Geometry check sheet. Reference: the model listing, model coordinates, mm. A direction names the side the tool comes from. Round coordinates to 2 decimals unless told otherwise and drop trailing zeros. Write each loop counter-clockwise with the first axis right and the second up, starting at its lowest first coordinate (ties: lowest second). Pieces come first, ordered by that corner, then holes. Notation, with made-up numbers: (-28.5, 23) -> (22.5, 23) arc R17 cw to (22.5, 54) -> close; hole circle Ø2 at (16.25, 68.5). An arc over 180 degrees is marked (long way). One line per question, with ' | ' between items.
```python
from build123d import *

# Parameters (mm, degrees)
BASE_FLANGE1_DEPTH               = 266.7
F_10_0_1935_DIAMETER_HOLE1_D     = 4.9149
F_29_64_0_45313_DIAMETER_HOLE1_D = 11.509502
F_11_32_0_34375_DIAMETER_HOLE1_D = 8.73125
EDGE_FLANGE1_DEPTH               = 34.925
F_11_32_0_34375_DIAMETER_HOLE2_D = 8.73125
F_11_32_0_34375_DIAMETER_HOLE6_D = 8.73125
FILLET1_R                        = 3.175
F_10_0_1935_DIAMETER_HOLE2_D     = 4.9149


# Sheet-metal steps are written as plain solids
with BuildPart() as part:
    # Sketch1 → Base-Flange1 (new, symmetric)
    with BuildSketch(Plane(origin=(0, 0, 0), x_dir=(1, 0, 0), z_dir=(0, 1, 0))):
        with BuildLine():
            Line((38.1, 0), (3.175, 0))
            ThreePointArc((3.175, 0), (0.92993597, -0.92993597), (0, -3.175))
            Line((0, -3.175), (0, -38.1))
            Line((0, -38.1), (-3.175, -38.1))
            Line((-3.175, -38.1), (-3.175, -3.175))
            ThreePointArc((-3.175, -3.175), (-1.315128061, 1.315128061), (3.175, 3.175))
            Line((3.175, 3.175), (38.1, 3.175))
            Line((38.1, 3.175), (38.1, 0))
        make_face()
    extrude(amount=BASE_FLANGE1_DEPTH, both=True)

    # #10 (0.1935) Diameter Hole1 (through all)
    with Locations(Plane.XY):
        with Locations((20.6375, -196.85), (20.6375, 0), (20.6375, 196.85)):
            Hole(F_10_0_1935_DIAMETER_HOLE1_D / 2)

    # 29/64 (0.45313) Diameter Hole1 (through all)
    with Locations(Plane.XY):
        with Locations((17.4625, 247.904), (17.4625, 95.504), (17.4625, -56.896), (17.4625, -209.296)):
            Hole(F_29_64_0_45313_DIAMETER_HOLE1_D / 2)

    # 11/32 (0.34375) Diameter Hole1 (through all)
    with Locations(Plane.XY):
        with Locations((20.6375, 228.6), (20.6375, 76.2), (20.6375, -76.2), (20.6375, -228.6)):
            Hole(F_11_32_0_34375_DIAMETER_HOLE1_D / 2)

    # Edge-Flange1 section (across the edge) → Edge-Flange1 (add)
    with BuildSketch(Plane(origin=(0, 273.304, 3.175), x_dir=(0, -1, 0), z_dir=(0, 0, 1))):
        with BuildLine():
            Line((0, 3.175), (0, 38.1))
            Line((0, 38.1), (3.175, 38.1))
            Line((3.175, 38.1), (3.175, 3.175))
            ThreePointArc((3.175, 3.175), (4.10493597, 0.92993597), (6.35, 0))
            Line((6.35, 0), (6.604, 0))
            Line((6.604, 0), (6.604, -3.175))
            Line((6.604, -3.175), (6.35, -3.175))
            ThreePointArc((6.35, -3.175), (1.859871939, -1.315128061), (0, 3.175))
        make_face()
    extrude(amount=EDGE_FLANGE1_DEPTH)

    # 11/32 (0.34375) Diameter Hole2 (through all)
    with Locations(Plane(origin=(0, 0, 0), x_dir=(0, 0, -1), z_dir=(1, 0, 0))):
        with Locations((-20.6375, 228.854), (-20.6375, 76.369333333), (-20.6375, -76.115333333), (-20.6375, -228.6)):
            Hole(F_11_32_0_34375_DIAMETER_HOLE2_D / 2)

    # 11/32 (0.34375) Diameter Hole6 (through all)
    with Locations(Plane(origin=(0, 273.304, 0), x_dir=(1, 0, 0), z_dir=(0, 1, 0))):
        with Locations((20.6375, -20.6375)):
            Hole(F_11_32_0_34375_DIAMETER_HOLE6_D / 2)

    # Fillet1
    fillet1_edges = [part.edges().sort_by_distance(p)[0] for p in [
        (38.1, 271.7165, 3.175),
        (38.1, 271.7165, 38.1),
        (38.1, 266.7, -1.5875),
        (38.1, -266.7, -1.5875),
        (-1.5875, -266.7, 38.1),
    ]]
    fillet(fillet1_edges, radius=FILLET1_R)

    # #10 (0.1935) Diameter Hole2 (through all)
    with Locations(Plane(origin=(0, 0, 0), x_dir=(0, 0, -1), z_dir=(1, 0, 0))):
        with Locations((-20.6375, 197.104), (-20.6375, -196.85), (-20.6375, 0.127)):
            Hole(F_10_0_1935_DIAMETER_HOLE2_D / 2)


solid = part.part
```
(1) Sectioned sample at A-A on y = -228.6. Record the cut outline in (x, z) (3 decimals).
Resolved:
outline: (-3.175, 3.175) arc R6.35 ccw to (3.175, -3.175) -> (16.272, -3.175) -> (16.272, 0) -> (3.175, 0) arc R3.175 cw to (0, 3.175) -> (0, 16.272) -> (-3.175, 16.272) -> close; (-3.175, 25.003) -> (0, 25.003) -> (0, 38.1) -> (-3.175, 38.1) -> close; (25.003, -3.175) -> (38.1, -3.175) -> (38.1, 0) -> (25.003, 0) -> close
(2) Go/stop test with flat-tipped pins: pin 1 (1.5 mm diameter, centred on x = 19.5, z = 16.5, fed in from -Y); pin 2 (7 mm diameter, centred on x = 20.64, y = 76.2, fed in from +Z); pin 3 (4 mm diameter, centred on y = 52.5, z = 28, fed in from +X); pin 4 (3.5 mm diameter, centred on x = 24, y = 269.5, fed in from -Z) (3 decimals). Record where each tip stops, or that it passes through.
Resolved:
pin 1: stops at y = 270.13 | pin 2: passes through | pin 3: stops at x = 0 | pin 4: stops at z = 3.175
(3) Material ranges on line 1 (Y direction, x = 6.5, z = 22); line 2 (X direction, y = -218, z = 31.5) (3 decimals), recorded low to high.
Resolved:
line 1: y = 270.13 to 273.3 | line 2: x = -3.175 to 0
(4) Access from +Z, -Z, +X, -X, +Y, -Y to the whole of each face (thin tool, end or side, straight path). Record for faces 1 (the flat face through (-1, -266.7, 7)), 2 (the flat face through (0, 4, 20)).
Resolved:
face 1: +Z, -Z, +X, -X, -Y | face 2: +Z, +X, -Y
(5) Draft check along Y on faces 3 (the cylindrical face through (-1.61, 72.108, 19.691)), 4 (the flat face through (-1, 4, 38.1)), 5 (the flat face through (25, 270.129, 17)), 6 (the cylindrical face through (-1.61, 224.592, 19.691)). Enter one of: +Y half, -Y half, draft (parallel to the pull), parting line (faces both ways), or undercut.
Resolved:
face 3: undercut | face 4: draft | face 5: -Y half | face 6: undercut
